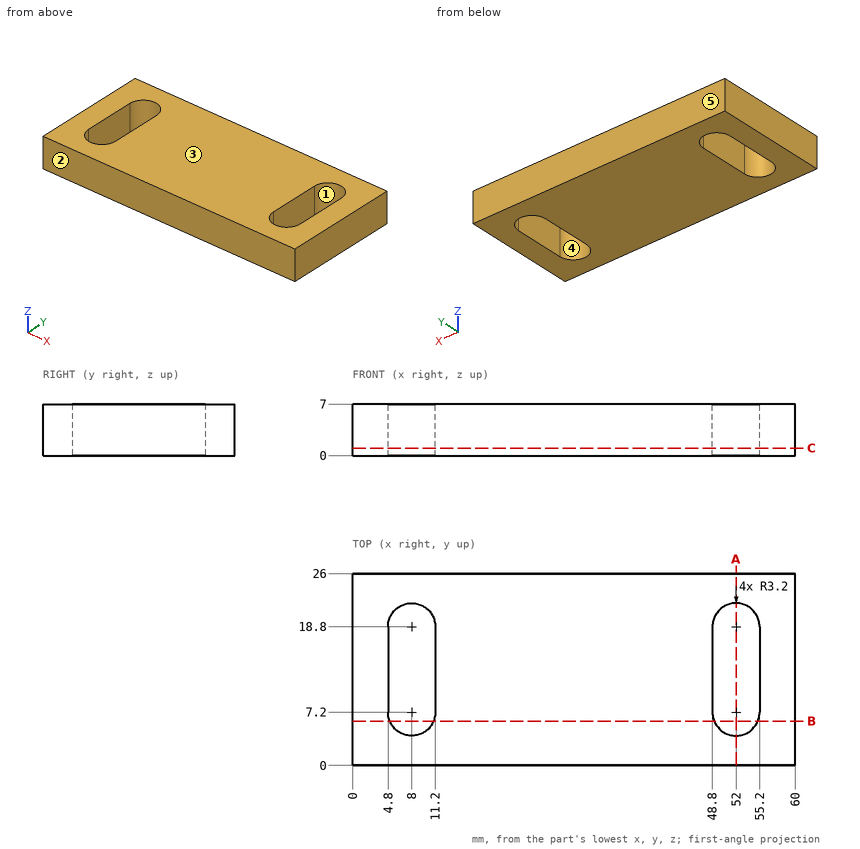
Source: three-view drawing plus pictorial views. Frame: mm from the lowest corner of the part. A direction names the side the tool comes from. Coordinates: 2 decimals unless noted, no trailing zeros. Loops run counter-clockwise (first coordinate to the right, second up) from the corner with the lowest first, then second, coordinate; pieces in that order, holes last. Notation, with made-up numbers: (43.25, -18) - (101.25, -18) arc R22 cw to (101.25, 0) - close; hole circle Ø5 at (28, -32.75). An arc over 180 degrees is marked (long way). Answer in a Markdown table with one row per item. Add a question column.
Item 1: Section query C-C on z = 1. Return the cut outline in (x, y).
Item 2: Mould query, pull axis Y, two halves, no side actions, for the marked faces 1, 2 and 3. Classes: released by +Y, released by -Y, zero draft, split by the parting line, or undercut.
Item 3: Line query: line 1 along X through (y, z) = (16.25, 3.5); line 2 along X through (y, z) = (4.5, 5); line 3 along Y through (x, z) = (8, 4.75). Output: solid intervals per line, ascending. Write a range as [from, to].
Item 4: Section query B-B on y = 6. Return the cut outline in (x, z), then the cut area to 3 significant figures.
Item 5: Section query A-A on x = 52. Return the cut outline in (y, z).
Item 6: Access query for the marked faces 4 and 5. Directions: +Z, -Z, +X, -X, +Y, -Y. A direction counts if a zero-diameter tool reaches every point of the face in a straight line with its end or side. Return the directions, or none.
Item 7: Contact query for a flat-ended pin moving along its axis: P1, Ø2, axis at y = 12.5, z = 3, coming from the -X side. Output: stop coordinate, or through.
Recorded:
| question | item | result |
|---|---|---|
| 1 | outline | (0, 0) - (60, 0) - (60, 26) - (0, 26) - close; hole (4.8, 7.2) arc R3.2 ccw to (11.2, 7.2) - (11.2, 18.8) arc R3.2 ccw to (4.8, 18.8) - close; hole (48.8, 7.2) arc R3.2 ccw to (55.2, 7.2) - (55.2, 18.8) arc R3.2 ccw to (48.8, 18.8) - close |
| 2 | face 1 | undercut |
| 2 | face 2 | released by -Y |
| 2 | face 3 | zero draft |
| 3 | line 1 | [0, 4.8], [11.2, 48.8], [55.2, 60] |
| 3 | line 2 | [0, 6.28], [9.72, 50.28], [53.72, 60] |
| 3 | line 3 | [0, 4], [22, 26] |
| 4 | outline | (0, 0) - (5.03, 0) - (5.03, 7) - (0, 7) - close; (10.97, 0) - (49.03, 0) - (49.03, 7) - (10.97, 7) - close; (54.97, 0) - (60, 0) - (60, 7) - (54.97, 7) - close |
| 4 | area | 337 mm^2 |
| 5 | outline | (0, 0) - (4, 0) - (4, 7) - (0, 7) - close; (22, 0) - (26, 0) - (26, 7) - (22, 7) - close |
| 6 | face 4 | +Z, -Z |
| 6 | face 5 | +Z, -Z, +X, -X, +Y |
| 7 | P1 | x = 0 |
